from build123d import *

# Parameters (mm, degrees)
F0_W     = 4
F0_H     = 5
F1_DEPTH = 3
F0_W_2   = 5
F0_W_3   = 70
F0_H_2   = 4.5
F2_DEPTH = 2
F3_D     = 2.5
F4_F1_R  = 1
F4_F2_R  = 1


with BuildPart() as f1:
    # F0 (on Top) → F1 (new body)
    with BuildSketch(Plane.XY):
        Polygon((-35, -10), (35, -10), (35, -2.5), (30, -2.5), (30, 2.5), (35, 2.5), (35, 10), (-35, 10), (-35, 2.5), (-30, 2.5), (-30, -2.5), (-35, -2.5), align=None)
        with Locations((-17.5, 0)):
            Rectangle(F0_W, F0_H, mode=Mode.SUBTRACT)
        with Locations((17.5, 0)):
            Rectangle(F0_W, F0_H, mode=Mode.SUBTRACT)
    extrude(amount=F1_DEPTH)

    # F0 (on Top) → F2 (join)
    with BuildSketch(Plane.XY):
        with Locations((-32.5, 0)):
            Rectangle(F0_W_2, F0_H)
        with Locations((0, 12.25)):
            Rectangle(F0_W_3, F0_H_2)
        with Locations((0, -12.25)):
            Rectangle(F0_W_3, F0_H_2)
        with Locations((32.5, 0)):
            Rectangle(F0_W_2, F0_H)
    extrude(amount=F2_DEPTH)

    # F3 (through all)
    with Locations(Plane(origin=(0, 0, 0), x_dir=(1, 0, 0), z_dir=(0, 0, -1))):
        with Locations((-30, 12.5), (-30, -12.5), (30, -11.6784099489), (30, 12.5)):
            Hole(F3_D / 2)

    # F4: fillet of radius 1 on 12 edges, made by hand

    # F4_f1
    f4_f1_edges = [f1.edges().sort_by_distance(p)[0] for p in [
        (-19.5, 2.5, 1.5),
        (-15.5, 2.5, 1.5),
        (-15.5, -2.5, 1.5),
        (-19.5, -2.5, 1.5),
        (19.5, 2.5, 1.5),
        (19.5, -2.5, 1.5),
        (15.5, -2.5, 1.5),
        (15.5, 2.5, 1.5),
    ]]
    fillet(f4_f1_edges, radius=F4_F1_R)

    # F4_f2
    f4_f2_edges = [f1.edges().sort_by_distance(p)[0] for p in [
        (15.5, 0, 3),
        (-15.5, 0, 3),
        (-19.5, 0, 3),
        (19.5, 0, 3),
        (19.2071067812, 2.2071067812, 3),
        (19.2071067812, -2.2071067812, 3),
        (-19.2071067812, -2.2071067812, 3),
        (-19.2071067812, 2.2071067812, 3),
        (-15.7928932188, 2.2071067812, 3),
        (-15.7928932188, -2.2071067812, 3),
        (15.7928932188, -2.2071067812, 3),
        (15.7928932188, 2.2071067812, 3),
    ]]
    fillet(f4_f2_edges, radius=F4_F2_R)


solid = f1.part
Geometry: final body of the model. Coordinates: model frame, mm. A direction names the side the tool comes from. Coordinates: 2 decimals unless noted, no trailing zeros. Loops run counter-clockwise (first coordinate to the right, second up) from the corner with the lowest first, then second, coordinate; pieces in that order, holes last. Notation, with made-up numbers: M -21.5,53.25 L 3.5,53.25 A15 cw 3.5,69.25 Z; hole C 15.25,24.25 d1. An arc over 180 degrees is marked long. One line per item, written item: value. Start each with the question number.
1) Cut plane A-A (y = -12.5). Return loops of the section in (x, z).
2) Pin query (flat end, axial travel): P1, Ø1.1, axis at x = -33, z = 2.5, coming from the -Y side; P2, Ø0.8, axis at y = 0, z = 2.5, coming from the +X side; P3, Ø3, axis at x = 30, y = 11.68, coming from the +Z side; P4, Ø0.5, axis at x = 33, z = 2.5, coming from the +Y side. Return the tip coordinate at first contact, or that it passes through.
3) Material intervals for L1, parallel to X at y = -0.5, z = 0.2; L2, parallel to Y at x = -30, z = 0.85; L3, parallel to X at y = -12.5, z = 0.95, sorted ascending. Write a range as from..to.
4) Cut plane B-B (z = 1.5). Return loops of the section in (x, y).
5) Draft query along Y for faces 1 (the flat face through (-18, -2.5, 1)), 2 (the flat face through (0, -12, 2)), 3 (the flat face through (0, 14.5, 1)). Return one class per face: released by +Y, released by -Y, zero draft, split by the parting line, or undercut.
6) Reachability of faces 4 (the flat face through (15.5, 0, 1)), 5 (the flat face through (-33, 0, 2)), 6 (the flat face through (0, 12, 2)) from +Z, -Z, +X, -X, +Y, -Y: full face, straight path, thin tool, end or side. Return the list, or none.
Evaluation:
1. outline: M -35,0 L -31.25,0 L -31.25,2 L -35,2 Z; M -28.75,0 L 28.75,0 L 28.75,2 L -28.75,2 Z; M 31.25,0 L 35,0 L 35,2 L 31.25,2 Z
2. P1: y = -14.5
2. P2: x = 30
2. P3: z = 2
2. P4: y = 10
3. L1: -35..-19.5, -15.5..15.5, 19.5..35
3. L2: -14.5..-13.75, -11.25..11.25, 13.75..14.5
3. L3: -35..-31.25, -28.75..28.75, 31.25..35
4. outline: M -35,-14.5 L 35,-14.5 L 35,14.5 L -35,14.5 Z; hole C -30,-12.5 d2.5; hole C -30,12.5 d2.5; hole M -19.5,-1.5 A1 ccw -18.5,-2.5 L -16.5,-2.5 A1 ccw -15.5,-1.5 L -15.5,1.5 A1 ccw -16.5,2.5 L -18.5,2.5 A1 ccw -19.5,1.5 Z; hole M 15.5,-1.5 A1 ccw 16.5,-2.5 L 18.5,-2.5 A1 ccw 19.5,-1.5 L 19.5,1.5 A1 ccw 18.5,2.5 L 16.5,2.5 A1 ccw 15.5,1.5 Z; hole C 30,-12.5 d2.5; hole C 30,11.68 d2.5
5. face 1: undercut
5. face 2: zero draft
5. face 3: released by +Y
6. face 4: +Z, -Z
6. face 5: +Z, -X
6. face 6: +Z, +X, -X, +Y
